```python
from build123d import *

# Parameters (mm, degrees)
SKETCH_1_R          = 5.0528125
EXTRUDE_597_DEPTH   = 10.8
SKETCH_2_OUTSIDE_W  = 89.934
SKETCH_2_OUTSIDE_H  = 92.718
SKETCH_2_OUTSIDE_R  = 9
CUT_EXTRUDE_1_DEPTH = 18.482562741
CUT_EXTRUDE_1_DRAFT = -60
SKETCH_3_OUTSIDE_W  = 89.934
SKETCH_3_OUTSIDE_H  = 92.718
SKETCH_3_OUTSIDE_R  = 9
CUT_EXTRUDE_2_DEPTH = 18.482562741
CUT_EXTRUDE_2_DRAFT = -60


with BuildPart() as part:
    # 草图1 → Extrude 597 (new body)
    with BuildSketch(Plane.XY):
        Polygon((0, 10.392304845), (-9, 5.196152423), (-9, -5.196152423), (0, -10.392304845), (9, -5.196152423), (9, 5.196152423), align=None)
        with Locations(Location((0, 0, 0), (0, 0, 180))):
            Circle(SKETCH_1_R, mode=Mode.SUBTRACT)
    extrude(amount=EXTRUDE_597_DEPTH)


with BuildPart() as cut_extrude_1_tool:
    # 草图2 outside → 切除-拉伸1 (with draft: the straight prism first)
    with BuildSketch(Plane(origin=(0, 0, 0), x_dir=(-1, 0, 0), z_dir=(0, 0, -1))):
        Rectangle(SKETCH_2_OUTSIDE_W, SKETCH_2_OUTSIDE_H)
        Circle(SKETCH_2_OUTSIDE_R, mode=Mode.SUBTRACT)
    extrude(amount=-CUT_EXTRUDE_1_DEPTH)
    # 切除-拉伸1: the draft: its side faces are tilted about the plane it starts from
    cut_extrude_1_sides = [cut_extrude_1_tool.faces().sort_by_distance(p)[0] for p in [
        (0, -46.359, 9.241281371),
        (-44.967, 0, 9.241281371),
        (0, 46.359, 9.241281371),
        (44.967, 0, 9.241281371),
        (9, 0, 9.241281371),
    ]]
    draft(cut_extrude_1_sides, Plane(origin=(0, 0, 0), x_dir=(-1, 0, 0), z_dir=(0, 0, -1)), CUT_EXTRUDE_1_DRAFT)


with BuildPart() as part_1:
    add(part.part)

    # 切除-拉伸1: cut by cut_extrude_1_tool
    add(cut_extrude_1_tool.part, mode=Mode.SUBTRACT)


with BuildPart() as cut_extrude_2_tool:
    # 草图3 outside → 切除-拉伸2 (with draft: the straight prism first)
    with BuildSketch(Plane.XY.offset(10.8)):
        Rectangle(SKETCH_3_OUTSIDE_W, SKETCH_3_OUTSIDE_H)
        Circle(SKETCH_3_OUTSIDE_R, mode=Mode.SUBTRACT)
    extrude(amount=-CUT_EXTRUDE_2_DEPTH)
    # 切除-拉伸2: the draft: its side faces are tilted about the plane it starts from
    cut_extrude_2_sides = [cut_extrude_2_tool.faces().sort_by_distance(p)[0] for p in [
        (0, -46.359, 1.558718629),
        (44.967, 0, 1.558718629),
        (0, 46.359, 1.558718629),
        (-44.967, 0, 1.558718629),
        (-9, 0, 1.558718629),
    ]]
    draft(cut_extrude_2_sides, Plane.XY.offset(10.8), CUT_EXTRUDE_2_DRAFT)


with BuildPart() as part_2:
    add(part_1.part)

    # 切除-拉伸2: cut by cut_extrude_2_tool
    add(cut_extrude_2_tool.part, mode=Mode.SUBTRACT)


solid = part_2.part
```
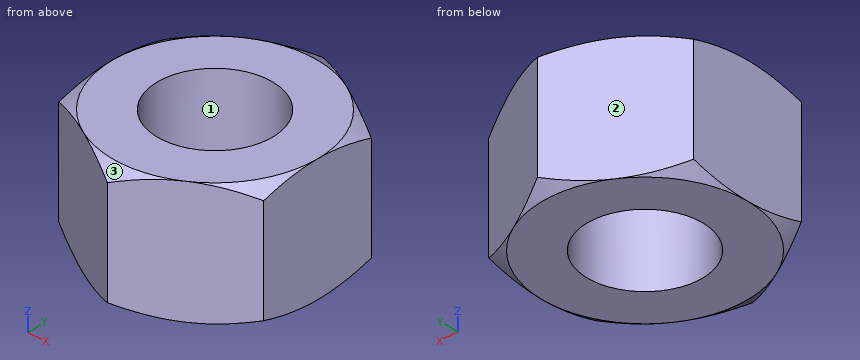
Work out the finished part from the listing and answer in its coordinate system (mm). Face numbers are marked on the shaded views. Give positions to 0.01 mm unless a question says otherwise; leave off trailing zeros. Loops run counter-clockwise (first coordinate to the right, second up) from the corner with the lowest first, then second, coordinate; pieces in that order, holes last. Notation, with made-up numbers: (-38, 11) -> (-7, 11) arc R17 ccw to (-7, 15) -> close; hole circle Ø5 at (59, -10). An arc over 180 degrees is marked (long way). Write item = value, one per line. Start each with the question number.
(1) Find section A-A on z = 6. Give the vertices of the cut face in (x, y), and give its area (3 significant figures).
(2) Find the intervals of material crossed by probe 1 along Y at (x, z) = (-1.5, 1.5); probe 2 along X at (y, z) = (-1, 5.5); probe 3 along X at (y, z) = (-3.5, 3), in increasing order. Write a range as from..to.
(3) The mould has two halves that part along Y. Classify the marked faces 1, 2 and 3: +Y half, -Y half, draft (parallel to the pull), parting line (faces both ways), or undercut.
(4) Given pin 1 Ø4 at (x, z) = (5.5, 5.5) entering from -Y; pin 2 Ø1 at (x, z) = (2.5, 6) entering from +Y; pin 3 Ø6 at (x, y) = (0, -7.5) entering from -Z, each flat-ended and moving along its own axis, determine where each tip first touches the part or whether it passes through.
From the geometry:
q1.outline = (-9, -5.2) -> (0, -10.39) -> (9, -5.2) -> (9, 5.2) -> (0, 10.39) -> (-9, 5.2) -> close; hole circle Ø10.11 at (0, 0)
q1.area = 200 mm^2
q2.probe_1 = -9.53..-4.83, 4.83..9.53
q2.probe_2 = -9..-4.95, 4.95..9
q2.probe_3 = -9..-3.64, 3.64..9
q3.face_1 = undercut
q3.face_2 = +Y half
q3.face_3 = -Y half
q4.pin_1 = -8.37
q4.pin_2 = 9.24
q4.pin_3 = 0
